Can you work these out from the model? Positions are in its coordinate system, mm. Face numbers are marked on the shaded views. A direction names the side the tool comes from. Coordinates: 2 decimals unless noted, no trailing zeros. Order: outer loops, then holes, each group sorted by start corner. A loop starts at its lowest first (then second) coordinate and runs counter-clockwise, first axis right, second up. Notation, with made-up numbers: (79.25, 77.25) -> (134.25, 77.25) arc R34 ccw to (134.25, 107.25) -> close; hole circle Ø5 at (15.5, 27). An arc over 180 degrees is marked (long way). Use a Markdown table: item, result. Add a question column.
1. Suppose I cut it at A-A, the plane z = 2.8. List the corners of the cut face in (x, y) for me.
2. For the marked faces 1, 2, 3 and 4, which set-ups out of +Z, -Z, +X, -X, +Y, -Y let a thin tool reach every point of the face, with its end or its side?
3. Suppose I cut it at D-D, the plane x = -1.75. List the corners of the cut face in (y, z) for me, then the cut area to 3 significant figures.
4. For pin 1 Ø1.5 at (x, z) = (-1, 2) entering from -Y; pin 2 Ø2 at (x, z) = (1, 1) entering from +Y; pin 3 Ø0.6 at (y, z) = (1.5, 2.5) entering from +X, each with a flat end and sliding along its axis, tell me the tip position at first contact or that it passes through.
5. Suppose I cut it at C-C, the plane x = 1. List the corners of the cut face in (y, z) for me.
6. If I drill on line 1 along X through (y, z) = (0, 3.5); line 2 along X through (y, z) = (0.5, 1.65); line 3 along Z through (x, y) = (-1, 0.75), over which ranges is the centre line in solid material (lowest first)? Write a range as from..to.
7. Suppose I cut it at B-B, the plane y = 0. List the corners of the cut face in (x, z) for me.
```python
from build123d import *

# Parameters (mm, degrees)
F0_R     = 3.5
F1_DEPTH = 0.5
F2_R     = 1.9
F2_R_2   = 1.4
F3_DEPTH = 3.2
F4_W     = 1
F4_H     = 6.460969
F5_DEPTH = 3.2


with BuildPart() as f1:
    # F0 (on Top) → F1 (new body, symmetric)
    with BuildSketch(Plane.XY):
        Circle(F0_R)
    extrude(amount=F1_DEPTH, both=True)

    # F2 (on face) → F3 (join)
    with BuildSketch(Plane.XY.offset(0.5)):
        Circle(F2_R)
        Circle(F2_R_2, mode=Mode.SUBTRACT)
    extrude(amount=F3_DEPTH)

    # F4 (on face) → F5 (cut, through all)
    with BuildSketch(Plane.XY.offset(3.7)):
        with Locations((0, -0.287181)):
            Rectangle(F4_W, F4_H)
    extrude(amount=-F5_DEPTH, mode=Mode.SUBTRACT)


solid = f1.part
```
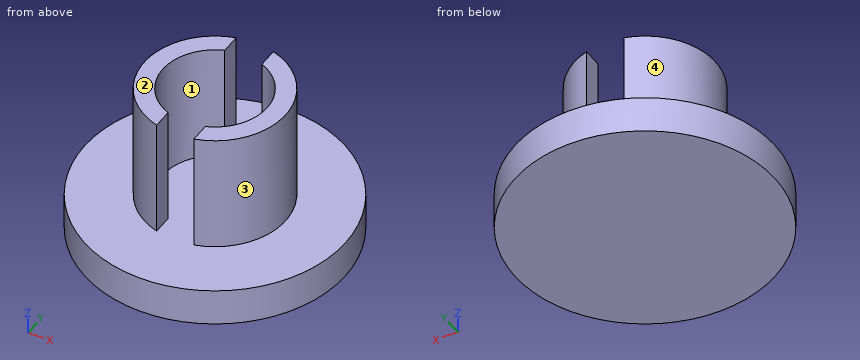
Worked out:
| question | item | result |
|---|---|---|
| 1 | outline | (-0.5, -1.83) -> (-0.5, -1.31) arc R1.4 cw to (-0.5, 1.31) -> (-0.5, 1.83) arc R1.9 ccw to start; (0.5, -1.83) arc R1.9 ccw to (0.5, 1.83) -> (0.5, 1.31) arc R1.4 cw to (0.5, -1.31) -> close |
| 2 | face 1 | +Z |
| 2 | face 2 | +Z, +X, -X, +Y, -Y |
| 2 | face 3 | +Z, +X |
| 2 | face 4 | +Z, -X |
| 3 | outline | (-3.03, -0.5) -> (3.03, -0.5) -> (3.03, 0.5) -> (0.74, 0.5) -> (0.74, 3.7) -> (-0.74, 3.7) -> (-0.74, 0.5) -> (-3.03, 0.5) -> close |
| 3 | area | 10.8 mm² |
| 4 | pin 1 | stops at y = -1.83 |
| 4 | pin 2 | stops at y = 3.5 |
| 4 | pin 3 | stops at x = 1.47 |
| 5 | outline | (-3.35, -0.5) -> (3.35, -0.5) -> (3.35, 0.5) -> (1.62, 0.5) -> (1.62, 3.7) -> (0.98, 3.7) -> (0.98, 0.5) -> (-0.98, 0.5) -> (-0.98, 3.7) -> (-1.62, 3.7) -> (-1.62, 0.5) -> (-3.35, 0.5) -> close |
| 6 | line 1 | x = -1.9..-1.4, 1.4..1.9 |
| 6 | line 2 | x = -1.83..-1.31, 1.31..1.83 |
| 6 | line 3 | z = -0.5..0.5 |
| 7 | outline | (-3.5, -0.5) -> (3.5, -0.5) -> (3.5, 0.5) -> (1.9, 0.5) -> (1.9, 3.7) -> (1.4, 3.7) -> (1.4, 0.5) -> (-1.4, 0.5) -> (-1.4, 3.7) -> (-1.9, 3.7) -> (-1.9, 0.5) -> (-3.5, 0.5) -> close |
